Can you work these out from the model? Positions are in its coordinate system, mm. A direction names the side the tool comes from. Coordinates: 2 decimals unless noted, no trailing zeros. Order: outer loops, then holes, each group sorted by start corner. A loop starts at its lowest first (then second) coordinate and runs counter-clockwise, first axis right, second up. Notation, with made-up numbers: (32, 46) -> (55, 46) arc R18 cw to (55, 73) -> close; hole circle Ø8 at (30, 27.5). An arc over 180 degrees is marked (long way). Answer in a Markdown table with one row per item. Add a question column.
1. On a 3-axis mill with a long thin cutter (end or side, diameter ignored), from which of +Z, -Z, +X, -X, +Y, -Y can I reach the whole of each face in a straight line? I mean faces 1 (the face through (0, 7.366, -12)), 2 (the face through (5.732, 24.088, -4.14)), 3 (the face through (6.75, 1.61, 7.27)). Say none if no direction works.
2. Imagine slicing it at B-B on y = 6.5. Write out the boundary of the cut face in (x, z).
3. We'd pull the mould along X, two halves only. Please class faces 4 (the face through (-2.744, 37.853, -8.715)), 5 (the face through (0, 30.861, -12)), 6 (the face through (-2.933, 17.897, -7.862)): pulls with the +X half, pulls with the -X half, needs draft (parallel to the pull), parting line crosses it, or undercut.
4. If I drill on line 1 along Y through (x, z) = (0, -7.75); line 2 along Y through (x, z) = (4, -8); line 3 along Y through (x, z) = (-6.5, 3.25), over which ranges is the centre line in solid material (lowest first)? Write a range as [from, to].
5. Will these pins go through, and if not, where does the flat tip stop? pin 1 (2 mm diameter, centred on x = -3, y = 14.5, fed in from +Z); pin 2 (2 mm diameter, centred on y = 34, z = 8.5, fed in from -X); pin 3 (1.2 mm diameter, centred on x = 5.77, z = 7.58, fed in from +Y).
6. Imagine slicing it at A-A on z = 0. Write out the boundary of the cut face in (x, y).
7. Imagine slicing it at C-C on y = 29. Write out the boundary of the cut face in (x, z), plus the area to 3 significant figures.
from build123d import *

# Parameters (mm, degrees)
SKETCH2_R                           = 13.97
BOSS_EXTRUDE1_DEPTH                 = 38.1
CHAMFER1_SIZE                       = 5.08
SKETCH5_R                           = 7.9375
CUT_EXTRUDE2_DEPTH                  = 1.27
SKETCH8_W                           = 3.81
SKETCH8_H                           = 23.495
CUT_EXTRUDE4_DEPTH                  = 12.7
SKETCH9_W                           = 12.7
SKETCH9_H                           = 0.508
CUT_EXTRUDE5_DEPTH                  = 9.525
F_1_2_0_5_DIAMETER_HOLE1_D          = 12.7
F_1_4_0_25_DIAMETER_HOLE1_REACH     = 49.213
F_1_4_0_25_DIAMETER_HOLE1_BORE_R    = 3.175
B_0_238_DIAMETER_HOLE1_D            = 6.0452
B_0_238_DIAMETER_HOLE1_DEPTH        = 3.81
B_0_238_DIAMETER_HOLE1_TIP          = 1.816161307
F_1_16_0_0625_DIAMETER_HOLE1_REACH  = 49.213
F_1_16_0_0625_DIAMETER_HOLE1_BORE_R = 0.79375
CUT_EXTRUDE6_START                  = -1.27
SKETCH21_R                          = 7.9375
CUT_EXTRUDE6_DEPTH                  = 1.27
F_8_32_TAPPED_HOLE1_D               = 3.4544
F_8_32_TAPPED_HOLE1_DEPTH           = 6.35
F_8_32_TAPPED_HOLE1_CSINK_D         = 4.318
F_8_32_TAPPED_HOLE1_CSINK_ANGLE     = 90
F_8_32_TAPPED_HOLE1_TIP             = 1.037806461


# Read off the part's stored shape, not the designer's step: M2.5x0.45 Tapped Hole1
with BuildPart() as part:
    # Sketch2 → Boss-Extrude1 (new body)
    with BuildSketch(Plane(origin=(0, 0, 0), x_dir=(1, 0, 0), z_dir=(0, 1, 0))):
        with Locations(Location((0, 0, 0), (0, 0, 90))):
            Circle(SKETCH2_R)
    extrude(amount=BOSS_EXTRUDE1_DEPTH)

    # Chamfer1
    chamfer1_edges = [part.edges().sort_by_distance(p)[0] for p in [
        (0, 38.1, 13.97),
    ]]
    chamfer(chamfer1_edges, length=CHAMFER1_SIZE)

    # Sketch5 → Cut-Extrude2 (cut)
    with BuildSketch(Plane(origin=(0, 38.1, 0), x_dir=(1, 0, 0), z_dir=(0, 1, 0))):
        with Locations(Location((0, 0, 0), (0, 0, 270))):
            Circle(SKETCH5_R)
    extrude(amount=-CUT_EXTRUDE2_DEPTH, mode=Mode.SUBTRACT)

    # Sketch8 → Cut-Extrude4 (cut, symmetric)
    with BuildSketch(Plane(origin=(0, 0, 0), x_dir=(0, 0, -1), z_dir=(1, 0, 0))):
        with Locations((12.065, 19.1135)):
            Rectangle(SKETCH8_W, SKETCH8_H)
    extrude(amount=CUT_EXTRUDE4_DEPTH, both=True, mode=Mode.SUBTRACT)

    # Sketch9 → Cut-Extrude5 (cut, symmetric)
    with BuildSketch(Plane(origin=(0, 0, 0), x_dir=(1, 0, 0), z_dir=(0, 1, 0))):
        with Locations((0, 13.97)):
            Rectangle(SKETCH9_W, SKETCH9_H)
    extrude(amount=CUT_EXTRUDE5_DEPTH, both=True, mode=Mode.SUBTRACT)

    # 1/2 (0.5) Diameter Hole1 (through all)
    with Locations(Plane(origin=(0, 0, 0), x_dir=(-1, 0, 0), z_dir=(0, -1, 0))):
        with Locations((0, 0)):
            Hole(F_1_2_0_5_DIAMETER_HOLE1_D / 2)

    # 1/4 (0.25) Diameter Hole1 bore → 1/4 (0.25) Diameter Hole1 (cut, up to next)
    with BuildSketch(Plane(origin=(0, 0, -10.16), x_dir=(-1, 0, 0), z_dir=(0, 0, -1)), mode=Mode.PRIVATE) as f_1_4_0_25_diameter_hole1_sk1:
        with Locations((0, 19.1135)):
            Circle(F_1_4_0_25_DIAMETER_HOLE1_BORE_R)
    f_1_4_0_25_diameter_hole1_tool1 = extrude(f_1_4_0_25_diameter_hole1_sk1.sketch, amount=-F_1_4_0_25_DIAMETER_HOLE1_REACH, mode=Mode.PRIVATE) & part.part
    add(f_1_4_0_25_diameter_hole1_tool1.solids().sort_by_distance((0, 19.1135, -10.16))[0], mode=Mode.SUBTRACT)

    # B (0.238) Diameter Hole1
    with Locations(Plane(origin=(0, 0, -10.16), x_dir=(-1, 0, 0), z_dir=(0, 0, -1))):
        with Locations((4.939140867, 24.052640867), (4.939140867, 14.174359133), (-4.939140867, 14.174359133), (-4.939140867, 24.052640867)):
            Hole(B_0_238_DIAMETER_HOLE1_D / 2, depth=B_0_238_DIAMETER_HOLE1_DEPTH)
            with Locations((0, 0, -(B_0_238_DIAMETER_HOLE1_DEPTH + B_0_238_DIAMETER_HOLE1_TIP / 2))):  # 118° drill point
                Cone(0, B_0_238_DIAMETER_HOLE1_D / 2, B_0_238_DIAMETER_HOLE1_TIP, mode=Mode.SUBTRACT)

    # 1/16 (0.0625) Diameter Hole1 bore → 1/16 (0.0625) Diameter Hole1 (cut, up to next)
    with BuildSketch(Plane(origin=(0, 0, -10.16), x_dir=(-1, 0, 0), z_dir=(0, 0, -1)), mode=Mode.PRIVATE) as f_1_16_0_0625_diameter_hole1_sk1:
        with Locations((4.939140867, 24.052640867)):
            Circle(F_1_16_0_0625_DIAMETER_HOLE1_BORE_R)
    f_1_16_0_0625_diameter_hole1_tool1 = extrude(f_1_16_0_0625_diameter_hole1_sk1.sketch, amount=-F_1_16_0_0625_DIAMETER_HOLE1_REACH, mode=Mode.PRIVATE) & part.part
    # 1/16 (0.0625) Diameter Hole1 bore → 1/16 (0.0625) Diameter Hole1 (cut, up to next)
    with BuildSketch(Plane(origin=(0, 0, -10.16), x_dir=(-1, 0, 0), z_dir=(0, 0, -1)), mode=Mode.PRIVATE) as f_1_16_0_0625_diameter_hole1_sk2:
        with Locations((4.939140867, 14.174359133)):
            Circle(F_1_16_0_0625_DIAMETER_HOLE1_BORE_R)
    f_1_16_0_0625_diameter_hole1_tool2 = extrude(f_1_16_0_0625_diameter_hole1_sk2.sketch, amount=-F_1_16_0_0625_DIAMETER_HOLE1_REACH, mode=Mode.PRIVATE) & part.part
    # 1/16 (0.0625) Diameter Hole1 bore → 1/16 (0.0625) Diameter Hole1 (cut, up to next)
    with BuildSketch(Plane(origin=(0, 0, -10.16), x_dir=(-1, 0, 0), z_dir=(0, 0, -1)), mode=Mode.PRIVATE) as f_1_16_0_0625_diameter_hole1_sk3:
        with Locations((-4.939140867, 14.174359133)):
            Circle(F_1_16_0_0625_DIAMETER_HOLE1_BORE_R)
    f_1_16_0_0625_diameter_hole1_tool3 = extrude(f_1_16_0_0625_diameter_hole1_sk3.sketch, amount=-F_1_16_0_0625_DIAMETER_HOLE1_REACH, mode=Mode.PRIVATE) & part.part
    # 1/16 (0.0625) Diameter Hole1 bore → 1/16 (0.0625) Diameter Hole1 (cut, up to next)
    with BuildSketch(Plane(origin=(0, 0, -10.16), x_dir=(-1, 0, 0), z_dir=(0, 0, -1)), mode=Mode.PRIVATE) as f_1_16_0_0625_diameter_hole1_sk4:
        with Locations((-4.939140867, 24.052640867)):
            Circle(F_1_16_0_0625_DIAMETER_HOLE1_BORE_R)
    f_1_16_0_0625_diameter_hole1_tool4 = extrude(f_1_16_0_0625_diameter_hole1_sk4.sketch, amount=-F_1_16_0_0625_DIAMETER_HOLE1_REACH, mode=Mode.PRIVATE) & part.part
    add(f_1_16_0_0625_diameter_hole1_tool1.solids().sort_by_distance((-4.939141, 24.052641, -10.16))[0], mode=Mode.SUBTRACT)
    add(f_1_16_0_0625_diameter_hole1_tool2.solids().sort_by_distance((-4.939141, 14.174359, -10.16))[0], mode=Mode.SUBTRACT)
    add(f_1_16_0_0625_diameter_hole1_tool3.solids().sort_by_distance((4.939141, 14.174359, -10.16))[0], mode=Mode.SUBTRACT)
    add(f_1_16_0_0625_diameter_hole1_tool4.solids().sort_by_distance((4.939141, 24.052641, -10.16))[0], mode=Mode.SUBTRACT)

    # Sketch21 → Cut-Extrude6 (cut)
    with BuildSketch(Plane.XZ.offset(CUT_EXTRUDE6_START)):
        with Locations(Location((0, 0, 0), (0, 0, 90))):
            Circle(SKETCH21_R)
    extrude(amount=CUT_EXTRUDE6_DEPTH, mode=Mode.SUBTRACT)

    # #8-32 Tapped Hole1
    with Locations(Plane(origin=(0, 0, -13.716), x_dir=(-1, 0, 0), z_dir=(0, 0, -1))):
        with Locations((0, 3.683)):
            CounterSinkHole(F_8_32_TAPPED_HOLE1_D / 2, F_8_32_TAPPED_HOLE1_CSINK_D / 2, depth=F_8_32_TAPPED_HOLE1_DEPTH, counter_sink_angle=F_8_32_TAPPED_HOLE1_CSINK_ANGLE)
            with Locations((0, 0, -(F_8_32_TAPPED_HOLE1_DEPTH + F_8_32_TAPPED_HOLE1_TIP / 2))):  # 118° drill point
                Cone(0, F_8_32_TAPPED_HOLE1_D / 2, F_8_32_TAPPED_HOLE1_TIP, mode=Mode.SUBTRACT)

    # M2.5x0.45 Tapped Hole1 outline → M2.5x0.45 Tapped Hole1 (revolve, cut)
    with BuildSketch(Plane(origin=(-5.772039513, 0, -7.576884905), x_dir=(1, 0, 0), z_dir=(0, 0, 1))):
        Polygon((1.025, 3.175), (0, 3.790882135), (0, 0), (1.025, 0), align=None)
    revolve(axis=Axis((-5.772039513, 0, -7.576884905), (0, 1, 0)), mode=Mode.SUBTRACT)

    # M2.5x0.45 Tapped Hole1 2 outline → M2.5x0.45 Tapped Hole1 2 (revolve, cut)
    with BuildSketch(Plane(origin=(5.772039513, 0, 7.576884905), x_dir=(1, 0, 0), z_dir=(0, 0, 1))):
        Polygon((1.025, 3.175), (0, 3.790882135), (0, 0), (1.025, 0), align=None)
    revolve(axis=Axis((5.772039513, 0, 7.576884905), (0, 1, 0)), mode=Mode.SUBTRACT)


solid = part.part
Answers follow:
| question | item | result |
|---|---|---|
| 1 | face 1 | -Z, +X, -X |
| 1 | face 2 | -Z |
| 1 | face 3 | -Y |
| 2 | outline | (-2.65, -13.72) -> (2.65, -13.72) arc R13.97 ccw (long way) to start; hole circle Ø12.7 at (0, 0) |
| 3 | face 4 | parting line crosses it |
| 3 | face 5 | needs draft |
| 3 | face 6 | undercut |
| 4 | line 1 | y = [1.27, 1.96], [5.41, 15.94], [22.29, 36.83] |
| 4 | line 2 | y = [0, 11.3], [17.05, 21.18], [26.93, 38.05] |
| 4 | line 3 | y = [1.27, 36.83] |
| 5 | pin 1 | stops at z = 13.83 |
| 5 | pin 2 | stops at x = -11.31 |
| 5 | pin 3 | stops at y = 38.06 |
| 6 | outline | (-13.97, 0) -> (-7.94, 0) -> (-7.94, 1.27) -> (-6.35, 1.27) -> (-6.35, 36.83) -> (-7.94, 36.83) -> (-7.94, 38.1) -> (-8.89, 38.1) -> (-13.97, 33.02) -> close; (6.35, 1.27) -> (7.94, 1.27) -> (7.94, 0) -> (13.97, 0) -> (13.97, 33.02) -> (8.89, 38.1) -> (7.94, 38.1) -> (7.94, 36.83) -> (6.35, 36.83) -> close |
| 7 | outline | (-9.59, -10.16) -> (9.59, -10.16) arc R13.97 ccw (long way) to start; hole circle Ø12.7 at (0, 0) |
| 7 | area | 436 mm² |
